CAD build for the part. Positions are in the model's coordinates, mm. A direction names the side the tool comes from. Round coordinates to 2 decimals unless told otherwise and drop trailing zeros. Loops run counter-clockwise (first coordinate to the right, second up) from the corner with the lowest first, then second, coordinate; pieces in that order, holes last. Notation, with made-up numbers: M 22.5,67 L 68.5,67 A13 cw 68.5,90 Z; hole C 47,10.5 d6. An arc over 180 degrees is marked long. Use a Markdown table: item, result. Add a question column.
(1) Band-saw the part on B-B, the plane y = -144.5. Write the cut outline in (x, z) (1 decimal).
(2) Band-saw the part on A-A, the plane z = 0. Write the cut outline in (x, y).
(3) Flat gauge pins, fed straight in: P1, Ø8, axis at x = -1.5, y = -109, coming from the -Z side; P2, Ø8, axis at x = -0.5, y = -67, coming from the +Z side; P3, Ø4, axis at y = -27.5, z = -2.5, coming from the -X side. Where does each tip first touch, or does it go through?
(4) Which spindle directions (+Z, -Z, +X, -X, +Y, -Y) get a long thin tool onto all of the face, cutting with end or side? Do faces 1 (the face through (-3, -5.687, -4)), 2 (the face through (3.522, -2.803, -6.216)). Say none if no direction does.
(5) Wall check: L1, parallel to X at y = -54, z = 0.5; L2, parallel to Y at x = 4.5, z = 5.25; L3, parallel to X at y = -82, z = 0.25. Give the ranges that are in metal, low to high.
from build123d import *

# Parameters (mm, degrees)
F0_R     = 4.7625
F1_DEPTH = 185.33872
F2_DEPTH = 5.6865671642


# Not quite as in the source:
# - a length typed as a fraction of an inch, garbled in the dataset ("3 / 203.2 mm" for 3/8 in), is restored


with BuildPart() as f1:
    # F0 (on Front) → F1 (new body)
    with BuildSketch(Plane.XZ):
        Circle(F0_R)
    extrude(amount=F1_DEPTH)

    # F0 (on Front) → F2 (join)
    with BuildSketch(Plane.XZ):
        Polygon((7.14375, -4.1244459855), (7.14375, 4.1244459855), (0, 8.248891971), (-7.14375, 4.1244459855), (-7.14375, -4.1244459855), (0, -8.248891971), align=None)
        Circle(F0_R, mode=Mode.SUBTRACT)
    extrude(amount=F2_DEPTH)


solid = f1.part
Return value:
| question | item | result |
|---|---|---|
| 1 | outline | C 0,0 d9.5 |
| 2 | outline | M -7.14,-5.69 L -4.76,-5.69 L -4.76,-185.34 L 4.76,-185.34 L 4.76,-5.69 L 7.14,-5.69 L 7.14,0 L -7.14,0 Z |
| 3 | P1 | z = -4.76 |
| 3 | P2 | z = 4.76 |
| 3 | P3 | x = -4.74 |
| 4 | face 1 | -Y |
| 4 | face 2 | -Z, +X, +Y, -Y |
| 5 | L1 | -4.74 to 4.74 |
| 5 | L2 | -5.69 to 0 |
| 5 | L3 | -4.76 to 4.76 |
